from build123d import *

# Parameters (mm, degrees)
MODEL_R             = 1.575000001
MODEL_R_2           = 3.05
MODEL_R_3           = 9.000000001
BOSS_EXTRUDE1_DEPTH = 3.175


with BuildPart() as part:
    # Model → Boss-Extrude1 (new body)
    with BuildSketch(Plane.XY):
        with BuildLine():
            Line((-57.393758137, 42.970698671), (-21.353966815, 7.026278384))
            ThreePointArc((-21.353966815, 7.026278384), (-22.382377018, 0.28718893), (-21.353966815, -6.451900523))
            Line((-21.353966815, -6.451900523), (-57.393758137, -42.39632081))
            ThreePointArc((-57.393758137, -42.39632081), (-57.413974609, -57.655322639), (-42.15497278, -57.675539111))
            Line((-42.15497278, -57.675539111), (-5.859634798, -21.47624841))
            ThreePointArc((-5.859634798, -21.47624841), (0.212184024, -22.307372111), (6.284002846, -21.47624841))
            Line((6.284002846, -21.47624841), (42.579340828, -57.675539111))
            ThreePointArc((42.579340828, -57.675539111), (57.838342657, -57.655322639), (57.818126185, -42.39632081))
            Line((57.818126185, -42.39632081), (21.778334863, -6.451900523))
            ThreePointArc((21.778334863, -6.451900523), (22.806745065, 0.28718893), (21.778334863, 7.026278384))
            Line((21.778334863, 7.026278384), (57.818126185, 42.970698671))
            ThreePointArc((57.818126185, 42.970698671), (57.838342657, 58.229700499), (42.579340828, 58.249916972))
            Line((42.579340828, 58.249916972), (6.284002846, 22.05062627))
            ThreePointArc((6.284002846, 22.05062627), (0.212184024, 22.881749972), (-5.859634798, 22.05062627))
            Line((-5.859634798, 22.05062627), (-42.15497278, 58.249916972))
            ThreePointArc((-42.15497278, 58.249916972), (-57.413974609, 58.229700499), (-57.393758137, 42.970698671))
        make_face()
        with Locations((0, 15)):
            Circle(MODEL_R, mode=Mode.SUBTRACT)
        with Locations((-49.72265974, 49.752211816)):
            Circle(MODEL_R_2, mode=Mode.SUBTRACT)
        with Locations(Location((50.062895685, 49.995974034, 0), (0, 0, 180))):
            Circle(MODEL_R_2, mode=Mode.SUBTRACT)
        with Locations((50.250439225, -50.894025966)):
            Circle(MODEL_R_2, mode=Mode.SUBTRACT)
        with Locations(Location((-49.534886134, -51.141545777, 0), (0, 0, 180))):
            Circle(MODEL_R_2, mode=Mode.SUBTRACT)
        with Locations((-12.99, 7.5)):
            Circle(MODEL_R, mode=Mode.SUBTRACT)
        with Locations(Location((12.99, 7.5, 0), (0, 0, 180))):
            Circle(MODEL_R, mode=Mode.SUBTRACT)
        Circle(MODEL_R_3, mode=Mode.SUBTRACT)
        with Locations(Location((0, -15, 0), (0, 0, 180))):
            Circle(MODEL_R, mode=Mode.SUBTRACT)
    extrude(amount=BOSS_EXTRUDE1_DEPTH)


solid = part.part
The listing builds one solid part. Answer for the finished solid, in the listing's coordinates (mm). A direction names the side the tool comes from. Round coordinates to 2 decimals unless told otherwise and drop trailing zeros. Order: outer loops, then holes, each group sorted by start corner. A loop starts at its lowest first (then second) coordinate and runs counter-clockwise, first axis right, second up. Notation, with made-up numbers: (36, 9.5) -> (84, 9.5) arc R9 cw to (84, 22.5) -> close; hole circle Ø3 at (12.25, 14.5). An arc over 180 degrees is marked (long way). One line per item, written item: value.
Item 1: For a pull along Y with two mould halves and no side action, classify faces 1 (the cylindrical face through (50.724, 52.973, 1.565)), 2 (the flat face through (24.686, 40.404, 1.565)), 3 (the flat face through (24.178, -39.322, 1.565)) as released by +Y, released by -Y, zero draft, split by the parting line, or undercut.
Taken from the geometry:
face 1: undercut
face 2: released by +Y
face 3: released by -Y
Item 2: Find section D-D, the plane z = 0.55. State how many separate pieces and enclosed holes the cut face has, then the cut area to 3 significant figures.
Taken from the geometry:
separate pieces: 1
enclosed holes: 9
area: 6,180 mm2
Item 3: Find section A-A, the plane y = -15. Give the vertices of the cut face in (x, z) (3 decimals), then the cut area to 3 significant figures.
Taken from the geometry:
outline: (-29.925, 0) -> (-1.575, 0) -> (-1.575, 3.175) -> (-29.925, 3.175) -> close; (1.575, 0) -> (30.349, 0) -> (30.349, 3.175) -> (1.575, 3.175) -> close
area: 181 mm2
Item 4: Straight lines are drawn through the part: L1, parallel to Y at x = 0, z = 2 (3 decimals); L2, parallel to Y at x = -1, z = 0.25; L3, parallel to Y at x = -28, z = 0.15. For each, find the intervals that lie inside material, in ascending order.
Taken from the geometry:
L1: y = -22.306 to -16.575, -13.425 to -9, 9 to 13.425, 16.575 to 22.881
L2: y = -22.27 to -16.22, -13.78 to -8.94, 8.94 to 13.78, 16.22 to 22.85
L3: y = -43.56 to -13.08, 13.65 to 44.13
Item 5: For faces 4 (the flat face through (40.051, -24.676, 1.565)), 5 (the flat face through (-39.626, 25.25, 1.565)), 6 (the cylindrical face through (-57.58, -57.485, 1.565)), determine the directions among +Z, -Z, +X, -X, +Y, -Y from which every point of the face is accessible in a straight line to the end or side of a thin tool.
Taken from the geometry:
face 4: +Z, -Z, +X
face 5: +Z, -Z, -X
face 6: +Z, -Z
Item 6: Find section C-C, the plane x = 27. Give the vertices of the cut face in (y, z) (3 decimals).
Taken from the geometry:
outline: (-42.137, 0) -> (-11.66, 0) -> (-11.66, 3.175) -> (-42.137, 3.175) -> close; (12.234, 0) -> (42.712, 0) -> (42.712, 3.175) -> (12.234, 3.175) -> close
Item 7: Find section B-B, the plane x = 0. Give the vertices of the cut face in (y, z) (3 decimals).
Taken from the geometry:
outline: (-22.306, 0) -> (-16.575, 0) -> (-16.575, 3.175) -> (-22.306, 3.175) -> close; (-13.425, 0) -> (-9, 0) -> (-9, 3.175) -> (-13.425, 3.175) -> close; (9, 0) -> (13.425, 0) -> (13.425, 3.175) -> (9, 3.175) -> close; (16.575, 0) -> (22.881, 0) -> (22.881, 3.175) -> (16.575, 3.175) -> close
